from build123d import *

# Parameters (mm, degrees)
CROQUIS1_W              = 50
CROQUIS1_H              = 10
SALIENTE_EXTRUIR1_DEPTH = 2.5
CORTAR_EXTRUIR1_DEPTH   = 52.23475383
SALIENTE_EXTRUIR2_DEPTH = 5
SALIENTE_EXTRUIR3_DEPTH = 5


with BuildPart() as part:
    # Croquis1 → Saliente-Extruir1 (new, symmetric)
    with BuildSketch(Plane(origin=(0, 0, 0), x_dir=(1, 0, 0), z_dir=(0, 1, 0))):
        with Locations((25, 5)):
            Rectangle(CROQUIS1_W, CROQUIS1_H)
    extrude(amount=SALIENTE_EXTRUIR1_DEPTH, both=True)

    # Croquis2 → Cortar-Extruir1 (cut, through all)
    with BuildSketch(Plane(origin=(0, 2.5, 0), x_dir=(1, 0, 0), z_dir=(0, 1, 0))):
        with BuildLine():
            Line((50, 7.5), (37, 7.5))
            ThreePointArc((37, 7.5), (35.585786438, 6.914213562), (35, 5.5))
            Line((35, 5.5), (35, 4.5))
            ThreePointArc((35, 4.5), (35.585786438, 3.085786438), (37, 2.5))
            Line((37, 2.5), (50, 2.5))
            Line((50, 2.5), (50, 7.5))
        make_face()
    extrude(amount=-CORTAR_EXTRUIR1_DEPTH, mode=Mode.SUBTRACT)

    # Croquis3 → Saliente-Extruir2 (add)
    with BuildSketch(Plane(origin=(0, 2.5, 0), x_dir=(1, 0, 0), z_dir=(0, 1, 0))):
        with BuildLine():
            Line((0, 2.5), (-13, 2.5))
            ThreePointArc((-13, 2.5), (-14.414213562, 3.085786438), (-15, 4.5))
            Line((-15, 4.5), (-15, 5.5))
            ThreePointArc((-15, 5.5), (-14.414213562, 6.914213562), (-13, 7.5))
            Line((-13, 7.5), (0, 7.5))
            Line((0, 7.5), (0, 2.5))
        make_face()
    extrude(amount=-SALIENTE_EXTRUIR2_DEPTH)

    # Croquis4 → Saliente-Extruir3 (add)
    with BuildSketch(Plane(origin=(0, 2.5, 0), x_dir=(1, 0, 0), z_dir=(0, 1, 0))):
        with BuildLine():
            Line((17, 37.5), (18, 37.5))
            ThreePointArc((18, 37.5), (19.414213562, 36.914213562), (20, 35.5))
            Line((20, 35.5), (20, 22.5))
            Line((20, 22.5), (22.5, 22.5))
            Line((22.5, 22.5), (22.5, -27.5))
            Line((22.5, -27.5), (20, -27.5))
            Line((20, -27.5), (20, -14.5))
            ThreePointArc((20, -14.5), (19.414213562, -13.085786438), (18, -12.5))
            Line((18, -12.5), (17, -12.5))
            ThreePointArc((17, -12.5), (15.585786438, -13.085786438), (15, -14.5))
            Line((15, -14.5), (15, -27.5))
            Line((15, -27.5), (12.5, -27.5))
            Line((12.5, -27.5), (12.5, 22.5))
            Line((12.5, 22.5), (15, 22.5))
            Line((15, 22.5), (15, 35.5))
            ThreePointArc((15, 35.5), (15.585786438, 36.914213562), (17, 37.5))
        make_face()
    extrude(amount=-SALIENTE_EXTRUIR3_DEPTH)


solid = part.part
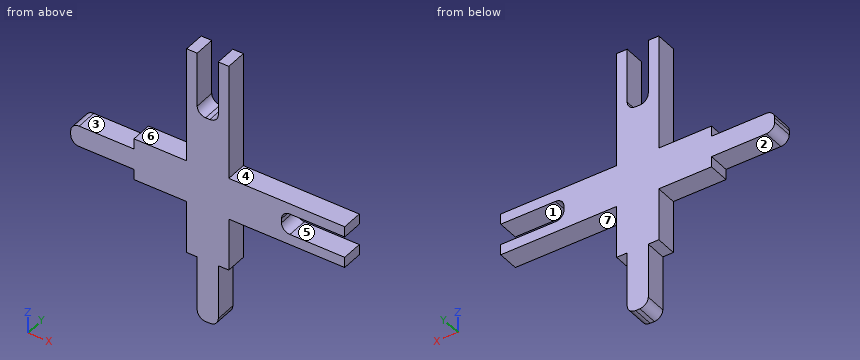
For this review, take the finished solid that the model builds, in its own axes (mm). Face numbers are marked on the shaded views. A direction names the side the tool comes from. Round coordinates to 2 decimals unless told otherwise and drop trailing zeros. Write each loop counter-clockwise with the first axis right and the second up, starting at its lowest first coordinate (ties: lowest second). Pieces come first, ordered by that corner, then holes. Notation, with made-up numbers: (49.5, -8.5) - (96.5, -8.5) arc R23 ccw to (96.5, 14.5) - close; hole circle Ø8 at (-25, 77.5). An arc over 180 degrees is marked (long way). Write item = value, one per line. Start each with the question number.
1. Consider section A-A on z = 23.5. State the section outline as (x, y) points.
2. Wall thickness on L1, parallel to Z at x = 40.5, y = 2; L2, parallel to X at y = -1.8, z = 15.5; L3, parallel to X at y = -0.55, z = -15: over which ranges is each line inside the solid? List them lowest first.
3. For pin 1 Ø1 at (y, z) = (1.5, 17) entering from -X; pin 2 Ø2 at (x, y) = (-5.5, -1.5) entering from +Z; pin 3 Ø1.2 at (y, z) = (1, -9) entering from -X; pin 4 Ø8 at (x, z) = (28.5, -25.5) entering from +Y, all flat-tipped, find the tip position at first contact; note any pin that passes through.
4. For the marked faces 1, 2, 3 and 4, list the 3-axis set-ups (+Z, -Z, +X, -X, +Y, -Y) from which the entire face can be reached by the end or side of a thin tool; tool diameter is ignored.
5. Draft analysis for pull direction Z (two halves, no side actions). For the marked faces 5, 6 and 7, state which applies: released by +Z, released by -Z, zero draft, split by the parting line, or undercut.
6. Consider section B-B on x = -9.5. State the section outline as (y, z) points, plus the area to 3 significant figures.
7. Consider section C-C on z = -9. State the section outline as (x, y) points.
Evaluation:
q1.outline = (12.5, -2.5) - (15, -2.5) - (15, 2.5) - (12.5, 2.5) - close; (20, -2.5) - (22.5, -2.5) - (22.5, 2.5) - (20, 2.5) - close
q2.L1 = -10 to -7.5, -2.5 to 0
q2.L2 = 12.5 to 15, 20 to 22.5
q2.L3 = 12.5 to 22.5
q3.pin_1 = 12.5
q3.pin_2 = -2.5
q3.pin_3 = 0
q3.pin_4 = through
q4.face_1 = +X, +Y, -Y
q4.face_2 = -Z, -X, +Y, -Y
q4.face_3 = +Z, -X, +Y, -Y
q4.face_4 = +Z, +X, +Y, -Y
q5.face_5 = undercut
q5.face_6 = released by +Z
q5.face_7 = released by -Z
q6.outline = (-2.5, -7.5) - (2.5, -7.5) - (2.5, -2.5) - (-2.5, -2.5) - close
q6.area = 25.0 mm2
q7.outline = (0, -2.5) - (50, -2.5) - (50, 2.5) - (0, 2.5) - close
